Autodesk Inventor part; units mm, degrees
ref_plane "YZ Plane" through (0, 0, 0) normal (1, 0, 0) x (0, 1, 0)
ref_plane "XZ Plane" through (0, 0, 0) normal (0, 1, 0) x (-1, 0, 0)
ref_plane "XY Plane" through (0, 0, 0) normal (0, 0, 1) x (1, 0, 0)
sketch "スケッチ1" plane through (0, 0, 0) normal (0, 0, 1) x (1, 0, 0)
  circle A0 centre (0, 0) radius 25
  circle A1 centre (0, 0) radius 6.15
  circle A2 centre (0, 0) radius 12.5
  line L0 (0, 0) -> (-8.8388, 8.8388)
  line L1 (0, 0) -> (12.5, 0) construction
  line L2 (-8.1009, 8.1009) -> (-4.5654, 11.6365)
  line L3 (-8.1009, 8.1009) -> (-11.6365, 4.5654)
  line L4 (8.1009, -8.1009) -> (4.5654, -11.6365)
  line L5 (8.1009, -8.1009) -> (11.6365, -4.5654)
  circle A3 centre (0, 18) radius 2.1
  circle A4 centre (-18, 0) radius 2.1
  circle A5 centre (0, -18) radius 2.1
  circle A6 centre (18, 0) radius 2.1
  dimension "d0" = 50
  dimension "d1" = 12.3
  dimension "d2" = 25
  dimension "d3" = 135
  dimension "d4" = 5
  dimension "d7" = 360
  dimension "d9" = 18
  dimension "d12" = 360
  dimension "d14" = 4.2
  dimension "d17" = 360
extrude "押し出し1" add sketch "スケッチ1" along normal blind 7 contours A0 | L2 L0 A2 | A2 L4 L5 | L0 L3 A2
extrude "押し出し2" add sketch "スケッチ1" along normal blind 20 contours A2 L5 L4 L3 L2
sketch "スケッチ2" plane through (11.6365, -4.5654, 20) normal (0.7071068, -0.7071068, 0) x (-0.7071068, -0.7071068, 0)
  line L0 (10, 0) -> (0, 0)
  point P0 (5, 20)
  point P1 (5, 6.5)
  dimension "d23" = 6.5
hole "穴1" at (8.1009, -8.1009, 13.5) direction (-0.7071068, 0.7071068, 0) diameter 4 end through all
properties part number "TH22_3DP_roller_fixer_sn" material "ABS プラスチック"
Input: part model. Units: mm. Frame: model coordinates. Coordinates: 2 decimals unless noted, no trailing zeros. Write each loop counter-clockwise with the first axis right and the second up, starting at its lowest first coordinate (ties: lowest second). Pieces come first, ordered by that corner, then holes. Notation, with made-up numbers: M 37,57.5 L 85,57.5 A27 cw 85,93.5 Z; hole C 72,-28.75 d4. An arc over 180 degrees is marked long. Use one line per item in the form item = value.
Q1. Section C-C (z = 14). Return loops of the section in (x, y).
Answer below:
outline = M -11.64,4.57 A12.5 ccw 4.57,-11.64 L 6.73,-9.47 L 2.76,-5.5 A6.15 cw -5.5,2.76 L -9.47,6.73 Z; M -6.73,9.47 L -2.76,5.5 A6.15 cw 5.5,-2.76 L 9.47,-6.73 L 11.64,-4.57 A12.5 ccw -4.57,11.64 Z
Q2. First-contact query: pin 1 (5 mm diameter, centred on y = 3.5, z = 6.5, fed in from -X); pin 2 (4 mm diameter, centred on x = 18, y = 0, fed in from -Z); pin 3 (2 mm diameter, centred on y = 17.5, z = 4.5, fed in from +X); pin 4 (1.5 mm diameter, centred on x = 11.5, z = 4.5, fed in from -Y). Flat tips, straight axial feed; report the tip coordinate or a pass-through.
Answer below:
pin_1 = -24.98
pin_2 = through
pin_3 = 18.78
pin_4 = -22.57
Q3. Material intervals for probe 1 along Y at (x, z) = (0, 10.75); probe 2 along Z at (x, y) = (-9.5, 16); probe 3 along Y at (x, z) = (4, 7.75), sorted ascending. Write a range as from..to.
Answer below:
probe_1 = -12.5..-6.15, 6.15..12.5
probe_2 = 0..7
probe_3 = -11.84..-4.67, 4.67..11.84
Q4. Section A-A (y = 0). Return loops of the section in (x, z).
Answer below:
outline = M -25,0 L -20.1,0 L -20.1,7 L -25,7 Z; M -15.9,0 L -6.15,0 L -6.15,20 L -12.5,20 L -12.5,7 L -15.9,7 Z; M 6.15,0 L 15.9,0 L 15.9,7 L 12.5,7 L 12.5,20 L 6.15,20 Z; M 20.1,0 L 25,0 L 25,7 L 20.1,7 Z
Q5. Section D-D (z = 3.5). Return loops of the section in (x, y), plus the area to 3 significant figures.
Answer below:
outline = C 0,0 d50; hole C -18,0 d4.2; hole C 0,0 d12.3; hole C 0,-18 d4.2; hole C 0,18 d4.2; hole C 18,0 d4.2
area = 1,790 mm²
Q6. Draft query along Y for faces 1 (the face through (-5.3, 7, 15.1)), 2 (the face through (-6, 11, 7)), 3 (the face through (-8.694, -8.981, 13.409)). Return one class per face: released by +Y, released by -Y, zero draft, split by the parting line, or undercut.
Answer below:
face_1 = undercut
face_2 = zero draft
face_3 = split by the parting line
